Check sheet for the modelled part. Datum: model origin and axes. Units: mm. Coordinates: 2 decimals unless noted, no trailing zeros. Write each loop counter-clockwise with the first axis right and the second up, starting at its lowest first coordinate (ties: lowest second). Pieces come first, ordered by that corner, then holes. Notation, with made-up numbers: (-1, 81.5) - (37, 81.5) arc R20 ccw to (37, 114.5) - close; hole circle Ø11 at (77, 39). An arc over 180 degrees is marked (long way). Use one line per item in the form item = value. Start each with the question number.
1. Go/stop test with a flat-tipped pin: pin 1 Ø0.5 at (x, y) = (38, 0.5) entering from -Z. Record where the tip stops, or that it passes through.
2. Scan lines: line 1 along Z through (x, y) = (0, 0.5); line 2 along X through (y, z) = (0.7, -2.5); line 3 along X through (y, z) = (0.15, -13.5). Record each from-to range of solid material in increasing order.
3. Draft check along X on faces 1 (the face through (1, 1.6, 1)), 2 (the face through (36.74, 0.79, -35.93)), 3 (the face through (11.923, 0.789, 53.692)). Enter one of: +X half, -X half, draft (parallel to the pull), parting line (faces both ways), or undercut.
4. Cross-section at D-D on z = -29. Record the boundary of the cut face in (x, y), then the cut area to 3 significant figures.
5. Cross-section at C-C on y = 0.4. Give the number of separate pieces and of enclosed holes in the cut face, then the cut area to 3 significant figures.
6. Cross-section at B-B on z = -15. Record the boundary of the cut face in (x, y), then the cut area to 3 significant figures.
7. Cross-section at A-A on x = 0. Record the boundary of the cut face in (y, z).
Autodesk Inventor part; units mm, degrees
ref_plane "YZ Plane" through (0, 0, 0) normal (1, 0, 0) x (0, 1, 0)
ref_plane "XZ Plane" through (0, 0, 0) normal (0, 1, 0) x (-1, 0, 0)
ref_plane "XY Plane" through (0, 0, 0) normal (0, 0, 1) x (1, 0, 0)
sketch "Эскиз1" plane through (0, 0, 0) normal (0, 1, 0) x (-1, 0, 0)
  circle A0 centre (0, 0) radius 55
  line L0 (79.4555, 0) -> (-79.4555, 0)
  line L1 (0, -103.8803) -> (0, 88.3129)
  dimension "d0" = 110
extrude "Выдавливание1" add sketch "Эскиз1" along normal blind 1.6
sketch "Эскиз2" plane through (0, 0, 0) normal (0, -1, 0) x (1, 0, 0)
  circle A0 centre (0, 0) radius 55
  line L0 (0, -103.8803) -> (0, 88.3129)
  line L1 (-79.4555, 0) -> (79.4555, 0)
  line L2 (11.5, -13.3) -> (23, -13.3)
  line L3 (23, -13.3) -> (23, 13.3)
  line L4 (23, 13.3) -> (11.5, 13.3)
  line L5 (11.5, 13.3) -> (11.5, -13.3)
  line L6 (35, -20) -> (45, -20)
  line L7 (45, -20) -> (45, 20)
  line L8 (45, 20) -> (35, 20)
  line L9 (35, 20) -> (35, -20)
  line L10 (17.25, -13.3) -> (17.25, 13.3)
  circle A1 centre (17.25, -9) radius 1
  circle A2 centre (17.25, 9) radius 1
  line L11 (3, 6) -> (33, 6)
  line L12 (33, 6) -> (33, -6)
  line L13 (33, -6) -> (3, -6)
  line L14 (3, -6) -> (3, 6)
  line L15 (-11.5, -13.3) -> (-23, -13.3)
  line L16 (-23, -13.3) -> (-23, 13.3)
  line L17 (-23, 13.3) -> (-11.5, 13.3)
  line L18 (-11.5, 13.3) -> (-11.5, -13.3)
  line L19 (-35, -20) -> (-45, -20)
  line L20 (-45, -20) -> (-45, 20)
  line L21 (-45, 20) -> (-35, 20)
  line L22 (-35, 20) -> (-35, -20)
  line L23 (-17.25, -13.3) -> (-17.25, 13.3)
  circle A3 centre (-17.25, -9) radius 1
  circle A4 centre (-17.25, 9) radius 1
  line L24 (-3, 6) -> (-33, 6)
  line L25 (-33, 6) -> (-33, -6)
  line L26 (-33, -6) -> (-3, -6)
  line L27 (-3, -6) -> (-3, 6)
  circle A5 centre (0, 0) radius 50
  circle A6 centre (0, -50) radius 1.5
  circle A7 centre (50, 0) radius 1.5
  circle A8 centre (0, 50) radius 1.5
  circle A9 centre (-50, 0) radius 1.5
  circle A10 centre (35.3553, -35.3553) radius 1.5
  circle A11 centre (50, 0) radius 1.5
  circle A12 centre (35.3553, 35.3553) radius 1.5
  circle A13 centre (0, 50) radius 1.5
  circle A14 centre (-35.3553, 35.3553) radius 1.5
  circle A15 centre (-50, 0) radius 1.5
  circle A16 centre (-35.3553, -35.3553) radius 1.5
  dimension "d6" = 11.5
  dimension "d7" = 26.6
  dimension "d9" = 10
  dimension "d10" = 40
  dimension "d11" = 45
  dimension "d12" = 12
  dimension "d13" = 2
  dimension "d14" = 18
  dimension "d15" = 2
  dimension "d16" = 30
  dimension "d17" = 12
  dimension "d18" = 2
  dimension "d21" = 100
  dimension "d22" = 3
  dimension "d23" = 3
  dimension "d25" = 3
  dimension "d26" = 3
  dimension "d30" = 360
extrude "Выдавливание2" cut sketch "Эскиз2" against normal blind 1.6 contours A7 A5 L1 | L1 A5 A7 | A8 A5 L0 | L0 A5 A8 | A6 A5 L0 | L0 A5 A6 | A5 A7 L1 | L1 A7 A5 | A9 A5 L1 | L1 A5 A9 | A5 A8 L0 | L0 A8 A5 | A5 A6 L0 | L0 A6 A5 | A12 A5 | A5 A12 | A10 A5 | A5 A10 | A5 A9 L1 | L1 A9 A5 | A14 A5 | A5 A14 | A16 A5 | A5 A16 | L7 L6 L9 L1 | L1 L9 L8 L7 | L20 L21 L22 L1 | L1 L22 L19 L20 | A3 L23 | L23 A3 | A4 L23 | L23 A4 | A1 L10 | L10 A1 | A2 L10 | L10 A2
sketch "Эскиз3" plane through (0, 0, 0) normal (0, -1, 0) x (1, 0, 0)
  circle A0 centre (50, 0) radius 1.5
  circle A1 centre (-50, 0) radius 1.5
  circle A2 centre (-17.25, 9) radius 1
  line L0 (35, -20) -> (35, 20)
  line L1 (35, 20) -> (45, 20)
  line L2 (45, 20) -> (45, -20)
  line L3 (45, -20) -> (35, -20)
  line L4 (-35, -20) -> (-45, -20)
  line L5 (-45, -20) -> (-45, 20)
  line L6 (-45, 20) -> (-35, 20)
  line L7 (-35, 20) -> (-35, -20)
  circle A3 centre (-35.3553, 35.3553) radius 1.5
  circle A4 centre (35.3553, -35.3553) radius 1.5
  circle A5 centre (35.3553, 35.3553) radius 1.5
  circle A6 centre (-35.3553, -35.3553) radius 1.5
  circle A7 centre (17.25, 9) radius 1
  circle A8 centre (17.25, -9) radius 1
  circle A9 centre (-17.25, -9) radius 1
  circle A10 centre (0, 50) radius 1.5
  circle A11 centre (0, -50) radius 1.5
  circle A12 centre (0, 0) radius 55
  line L8 (-79.4555, 0) -> (79.4555, 0)
  line L9 (0, -103.8803) -> (0, 88.3129)
  circle A13 centre (0, 0) radius 50
  circle A14 centre (-35.3553, -35.3553) radius 1.5
  line L10 (23, 13.3) -> (11.5, 13.3)
  line L11 (-21.1, -39.0646) -> (21.1, -39.0646)
  line L12 (21.1, -39.0646) -> (21.1, 37.2354)
  line L13 (21.1, 37.2354) -> (-21.1, 37.2354)
  line L14 (-21.1, 37.2354) -> (-21.1, -39.0646)
  circle A15 centre (-11, -24) radius 1.5
  circle A16 centre (11, -24) radius 1.5
  circle A17 centre (11, 24) radius 1.5
  circle A18 centre (-11, 24) radius 1.5
  dimension "d34" = 76.3
  dimension "d35" = 42.2
  dimension "d37" = 3
  dimension "d38" = 3
  dimension "d39" = 3
  dimension "d40" = 3
  dimension "d42" = 22
  dimension "d43" = 48
extrude "Выдавливание3" cut sketch "Эскиз3" against normal blind 1.6 contours A15 | A16 | A17 | A18
sketch "Эскиз4" plane through (0, 1.6, 0) normal (0, 1, 0) x (1, 0, 0)
  circle A0 centre (-11, 24) radius 1.5
  circle A1 centre (11, 24) radius 1.5
  circle A2 centre (11, -24) radius 1.5
  circle A3 centre (11, 24) radius 1.5
  circle A4 centre (-11, -24) radius 1.5
  circle A5 centre (-11, 24) radius 1.5
  circle A6 centre (50, 0) radius 1.5
  circle A7 centre (-50, 0) radius 1.5
  circle A8 centre (-17.25, -9) radius 1
  line L0 (45, -20) -> (35, -20)
  line L1 (35, -20) -> (35, 20)
  line L2 (35, 20) -> (45, 20)
  line L3 (45, 20) -> (45, -20)
  line L4 (-45, -20) -> (-45, 20)
  line L5 (-45, 20) -> (-35, 20)
  line L6 (-35, 20) -> (-35, -20)
  line L7 (-35, -20) -> (-45, -20)
  circle A9 centre (-35.3553, -35.3553) radius 1.5
  circle A10 centre (35.3553, 35.3553) radius 1.5
  circle A11 centre (35.3553, -35.3553) radius 1.5
  circle A12 centre (-35.3553, 35.3553) radius 1.5
  circle A13 centre (17.25, -9) radius 1
  circle A14 centre (17.25, 9) radius 1
  circle A15 centre (-17.25, 9) radius 1
  circle A16 centre (0, -50) radius 1.5
  circle A17 centre (0, 50) radius 1.5
  circle A18 centre (0, 0) radius 55
  line L8 (0, 103.8803) -> (0, -88.3129)
  line L9 (-79.4555, 0) -> (79.4555, 0)
  circle A19 centre (6.75, 40) radius 1.15
  circle A20 centre (-6.75, 40) radius 1.15
  circle A21 centre (6.75, -40) radius 1.15
  circle A22 centre (-6.75, -40) radius 1.15
  dimension "d48" = 2.3
  dimension "d51" = 13.5
  dimension "d52" = 10
  dimension "d54" = 2.3
  dimension "d56" = 13.5
  dimension "d57" = 10
extrude "Выдавливание4" cut sketch "Эскиз4" against normal blind 10 contours A19 | A20 | A21 | A22
properties part number "pcbCase"
Final values:
q1.pin_1 = -40
q2.line_1 = -55 to -51.5, -48.5 to 48.5, 51.5 to 55
q2.line_2 = -54.94 to -45, -35 to 35, 45 to 54.94
q2.line_3 = -53.32 to -45, -35 to 35, 45 to 53.32
q3.face_1 = draft
q3.face_2 = undercut
q3.face_3 = parting line
q4.outline = (-46.73, 0) - (46.73, 0) - (46.73, 1.6) - (-46.73, 1.6) - close
q4.area = 150 mm²
q5.separate_pieces = 1
q5.enclosed_holes = 22
q5.area = 8,590 mm²
q6.outline = (-52.92, 0) - (-45, 0) - (-45, 1.6) - (-52.92, 1.6) - close; (-35, 0) - (35, 0) - (35, 1.6) - (-35, 1.6) - close; (45, 0) - (52.92, 0) - (52.92, 1.6) - (45, 1.6) - close
q6.area = 137 mm²
q7.outline = (0, -55) - (1.6, -55) - (1.6, -51.5) - (0, -51.5) - close; (0, -48.5) - (1.6, -48.5) - (1.6, 48.5) - (0, 48.5) - close; (0, 51.5) - (1.6, 51.5) - (1.6, 55) - (0, 55) - close
